Model file for the job. Use its own axes, mm. A direction names the side the tool comes from. Round coordinates to 2 decimals unless told otherwise and drop trailing zeros. Order: outer loops, then holes, each group sorted by start corner. A loop starts at its lowest first (then second) coordinate and runs counter-clockwise, first axis right, second up. Notation, with made-up numbers: (78.25, 68) - (131.25, 68) arc R21 cw to (131.25, 101) - close; hole circle Ø11 at (-19, 31). An arc over 180 degrees is marked (long way). Answer as CSV lines item,"result". Start each with the question number.
1. 3-axis set-ups, long thin cutter, end or side, ignore diameter. For faces 1 (the face through (-83, 2, 11)), 2 (the face through (-112, 2, 21.15)), 3 (the face through (115, 2, 6.15)), 4 (the face through (-114, 2, -16.15)): which of +Z, -Z, +X, -X, +Y, -Y reach the whole face in a straight line?
2. Band-saw the part on D-D on x = 74.5. List the corners of the cut face in (y, z), then the cut area to 3 significant figures.
3. Pin check, flat tips, straight feed: pin 1 Ø1.5 at (x, y) = (57.5, 1) entering from +Z; pin 2 Ø1.5 at (y, z) = (1.5, 13.5) entering from +X; pin 3 Ø2.5 at (y, z) = (3, 10) entering from -X. Stop position of each tip, or through.
4. Pull direction X, two halves, no side cores. Call faces 5 (the face through (-117, 2, 19)), 6 (the face through (-98, 2, -21.15)), 7 (the face through (-97, 2, 24)): released by +X, released by -X, zero draft, split by the parting line, or undercut.
5. Band-saw the part on C-C on y = 2.8. State how many separate pieces and enclosed holes the cut face has, then the cut area to 3 significant figures.
6. Band-saw the part on B-B on z = -8.5. List the corners of the cut face in (x, y).
7. Wall check: line 1 along X through (y, z) = (1.3, 8); line 2 along X through (y, z) = (1.55, -15); line 3 along X through (y, z) = (1.65, -8). Give the ranges that are in metal, low to high. Write a range as [from, to].
8. Band-saw the part on A-A on z = 11. List the corners of the cut face in (x, y), then the cut area to 4 significant figures.
```python
from build123d import *

# Parameters (mm, degrees)
SKETCH_1_W      = 5
SKETCH_1_H      = 10
EXTRUDE_1_DEPTH = 5


with BuildPart() as part:
    # 草图1 → 凸台-拉伸1 (new body)
    with BuildSketch(Plane(origin=(0, 0, 0), x_dir=(1, 0, 0), z_dir=(0, 1, 0))):
        with BuildLine():
            Line((-117, 21.15), (-77.52077205, 21.15))
            ThreePointArc((-77.52077205, 21.15), (-75.590849256, 20.446823461), (-74.565644083, 18.666932006))
            Line((-74.565644083, 18.666932006), (-72.434355917, 6.483067994))
            ThreePointArc((-72.434355917, 6.483067994), (-71.409150744, 4.703176539), (-69.47922795, 4))
            Line((-69.47922795, 4), (103.47922795, 4))
            ThreePointArc((103.47922795, 4), (105.409150744, 4.703176539), (106.434355917, 6.483067994))
            Line((106.434355917, 6.483067994), (108.565644083, 18.666932006))
            ThreePointArc((108.565644083, 18.666932006), (109.590849256, 20.446823461), (111.52077205, 21.15))
            Line((111.52077205, 21.15), (117, 21.15))
            Line((117, 21.15), (117, 16.15))
            Line((117, 16.15), (112, 16.15))
            Line((112, 16.15), (112, 6.15))
            Line((112, 6.15), (117, 6.15))
            Line((117, 6.15), (117, -6.15))
            Line((117, -6.15), (112, -6.15))
            Line((112, -6.15), (112, -16.15))
            Line((112, -16.15), (117, -16.15))
            Line((117, -16.15), (117, -21.15))
            Line((117, -21.15), (107, -21.15))
            Line((107, -21.15), (107, -26.15))
            Line((107, -26.15), (97, -26.15))
            Line((97, -26.15), (97, -21.15))
            Line((97, -21.15), (10, -21.15))
            Line((10, -21.15), (10, -26.15))
            Line((10, -26.15), (-10, -26.15))
            Line((-10, -26.15), (-10, -21.15))
            Line((-10, -21.15), (-97, -21.15))
            Line((-97, -21.15), (-97, -26.15))
            Line((-97, -26.15), (-107, -26.15))
            Line((-107, -26.15), (-107, -21.15))
            Line((-107, -21.15), (-117, -21.15))
            Line((-117, -21.15), (-117, -16.15))
            Line((-117, -16.15), (-112, -16.15))
            Line((-112, -16.15), (-112, -6.15))
            Line((-112, -6.15), (-117, -6.15))
            Line((-117, -6.15), (-117, 6.15))
            Line((-117, 6.15), (-112, 6.15))
            Line((-112, 6.15), (-112, 16.15))
            Line((-112, 16.15), (-117, 16.15))
            Line((-117, 16.15), (-117, 21.15))
        make_face()
        with Locations((-80.5, 11.15)):
            Rectangle(SKETCH_1_W, SKETCH_1_H, mode=Mode.SUBTRACT)
        with Locations((-80.5, -11.15)):
            Rectangle(SKETCH_1_W, SKETCH_1_H, mode=Mode.SUBTRACT)
    extrude(amount=EXTRUDE_1_DEPTH)


solid = part.part
```
Reply:
1,face 1,"+Y, -Y"
1,face 2,"+Z, -X, +Y, -Y"
1,face 3,"+X, +Y, -Y"
1,face 4,"-X, +Y, -Y"
2,outline,"(0, -4) - (5, -4) - (5, 21.15) - (0, 21.15) - close"
2,area,"126 mm2"
3,pin 1,"stops at z = 21.15"
3,pin 2,"stops at x = 112"
3,pin 3,"stops at x = -112"
4,face 5,"released by -X"
4,face 6,"zero draft"
4,face 7,"undercut"
5,separate pieces,"1"
5,enclosed holes,"2"
5,area,"6,690 mm2"
6,outline,"(-112, 0) - (-83, 0) - (-83, 5) - (-112, 5) - close; (-78, 0) - (-72.79, 0) - (-72.79, 5) - (-78, 5) - close; (106.79, 0) - (112, 0) - (112, 5) - (106.79, 5) - close"
7,line 1,"x = [-112, -83], [-78, 112]"
7,line 2,"x = [-112, -83], [-78, -73.92], [107.92, 112]"
7,line 3,"x = [-112, -83], [-78, -72.7], [106.7, 112]"
8,outline,"(-112, 0) - (-83, 0) - (-83, 5) - (-112, 5) - close; (-78, 0) - (112, 0) - (112, 5) - (-78, 5) - close"
8,area,"1,095 mm2"
